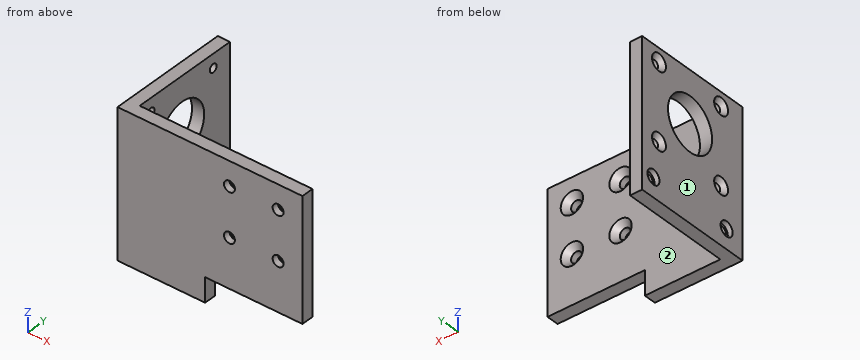
```python
from build123d import *

# Parameters (mm, degrees)
EXTRUDE_1_DEPTH             = 60
SKETCH_2_R                  = 11
CUT_EXTRUDE_1_DEPTH         = 60
CSK_1_D                     = 3.4
CSK_1_DEPTH                 = 5
CSK_1_CSINK_D               = 6.94
CSK_1_CSINK_ANGLE           = 90
SKETCH_5_W                  = 64
SKETCH_5_H                  = 10
CUT_EXTRUDE_2_DEPTH         = 127.885775404
SKETCH_6_R                  = 2
CUT_EXTRUDE_3_DEPTH         = 10
SKETCH_7_R                  = 3
CUT_EXTRUDE_4_DEPTH         = 2
SKETCH_8_W                  = 24
SKETCH_8_H                  = 50
CUT_EXTRUDE_5_DEPTH         = 127.885775404
HOLE_WIZARD_M41_D           = 4.5
HOLE_WIZARD_M41_CSINK_D     = 9.18
HOLE_WIZARD_M41_CSINK_ANGLE = 90


with BuildPart() as part:
    # Эскиз1 → Бобышка-Вытянуть1 (new body)
    with BuildSketch(Plane.XY):
        Polygon((0, 0), (0, 50), (5, 50), (5, 5), (95, 5), (95, 50), (100, 50), (100, 0), align=None)
    extrude(amount=EXTRUDE_1_DEPTH)

    # Эскиз2 → Вырез-Вытянуть1 (cut)
    with BuildSketch(Plane.ZY):
        with Locations((38.85, 26.15)):
            Circle(SKETCH_2_R)
    extrude(amount=-CUT_EXTRUDE_1_DEPTH, mode=Mode.SUBTRACT)

    # CSK размера винта с полупотайной головкой и крестообразным шлицем1
    with Locations(Plane.ZY):
        with Locations((54.35, 10.65), (54.35, 41.65), (23.35, 41.65), (23.35, 10.65)):
            CounterSinkHole(CSK_1_D / 2, CSK_1_CSINK_D / 2, depth=CSK_1_DEPTH, counter_sink_angle=CSK_1_CSINK_ANGLE)

    # Эскиз5 → Вырез-Вытянуть2 (cut, through all)
    with BuildSketch(Plane.XZ):
        with Locations((68, 5)):
            Rectangle(SKETCH_5_W, SKETCH_5_H)
    extrude(amount=-CUT_EXTRUDE_2_DEPTH, mode=Mode.SUBTRACT)

    # Эскиз6 → Вырез-Вытянуть3 (cut)
    with BuildSketch(Plane.ZY):
        with Locations((8, 44.4)):
            Circle(SKETCH_6_R)
        with Locations((8, 7.9)):
            Circle(SKETCH_6_R)
    extrude(amount=-CUT_EXTRUDE_3_DEPTH, mode=Mode.SUBTRACT)

    # Эскиз7 → Вырез-Вытянуть4 (cut)
    with BuildSketch(Plane.ZY):
        with Locations((8, 44.4)):
            Circle(SKETCH_7_R)
        with Locations((8, 7.9)):
            Circle(SKETCH_7_R)
    extrude(amount=-CUT_EXTRUDE_4_DEPTH, mode=Mode.SUBTRACT)

    # Эскиз8 → Вырез-Вытянуть5 (cut, through all)
    with BuildSketch(Plane.XZ):
        with Locations((88, 35)):
            Rectangle(SKETCH_8_W, SKETCH_8_H)
    extrude(amount=-CUT_EXTRUDE_5_DEPTH, mode=Mode.SUBTRACT)

    # Зенковка для винта с потайной головкой и внутренним шестигранником M41 (through all)
    with Locations(Plane(origin=(0, 5, 0), x_dir=(-1, 0, 0), z_dir=(0, 1, 0))):
        with Locations((-46, 30), (-66, 30), (-46, 50), (-66, 50)):
            CounterSinkHole(HOLE_WIZARD_M41_D / 2, HOLE_WIZARD_M41_CSINK_D / 2, counter_sink_angle=HOLE_WIZARD_M41_CSINK_ANGLE)


solid = part.part
```
Design review of the part built by this model. Coordinates are the model's own, in mm. Face numbers are marked on the shaded views. A direction names the side the tool comes from. Give positions to 0.01 mm unless a question says otherwise; leave off trailing zeros. Order: outer loops, then holes, each group sorted by start corner. A loop starts at its lowest first (then second) coordinate and runs counter-clockwise, first axis right, second up. Notation, with made-up numbers: (-23, 59) - (0, 59) arc R21 ccw to (0, 83) - close; hole circle Ø4 at (28.25, -24.75). An arc over 180 degrees is marked (long way). Use a Markdown table: item, result. Add a question column.
(1) Add section A-A on x = 66. Give the boundary of the cut face in (y, z).
(2) Add section C-C on z = 42. Give the boundary of the cut face in (x, y).
(3) Machinability: for the marked faces 1 and 2, which of the approach directions +Z, -Z, +X, -X, +Y, -Y give a long, thin tool a straight path to every point of the face, cutting with its end or side? Answer none if there is none.
(4) Wall thickness on probe 1 along Y at (x, z) = (1.2, 8); probe 2 along X at (y, z) = (2, 50); probe 3 along Y at (x, z) = (4.2, 8): over which ranges is each line inside the solid? List them lowest first. Write a range as [from, to].
(5) Add section B-B on z = 8. Give the boundary of the cut face in (x, y).
(6) Clearance check with flat-ended pins moving along their axes: P1, Ø17.5, axis at y = 26.15, z = 38.85, coming from the -X side; P2, Ø5, axis at y = 44.4, z = 8, coming from the +X side; P3, Ø4, axis at x = 24, z = 49.5, coming from the +Y side; P4, Ø3, axis at x = 65, z = 49.5, coming from the +Y side. State where each tip first meets the part, or that it passes through.
(7) Add section D-D on z = 17. Give the boundary of the cut face in (x, y).
Report:
| question | item | result |
|---|---|---|
| 1 | outline | (0, 10) - (5, 10) - (5, 25.41) - (2.66, 27.75) - (0, 27.75) - close; (0, 32.25) - (2.66, 32.25) - (5, 34.59) - (5, 45.41) - (2.66, 47.75) - (0, 47.75) - close; (0, 52.25) - (2.66, 52.25) - (5, 54.59) - (5, 60) - (0, 60) - close |
| 2 | outline | (0, 0) - (76, 0) - (76, 5) - (5, 5) - (5, 15.61) - (0, 15.61) - close; (0, 36.69) - (5, 36.69) - (5, 50) - (0, 50) - close |
| 3 | face 1 | +Z, -Z, -X, +Y, -Y |
| 3 | face 2 | +Z, -Z, +X, +Y |
| 4 | probe 1 | y = [0, 4.9], [10.9, 41.4], [47.4, 50] |
| 4 | probe 2 | x = [0, 43.75], [48.25, 63.75], [68.25, 76] |
| 4 | probe 3 | y = [0, 5.9], [9.9, 42.4], [46.4, 50] |
| 5 | outline | (0, 0) - (36, 0) - (36, 5) - (5, 5) - (5, 5.9) - (2, 5.9) - (2, 4.9) - (0, 4.9) - close; (0, 10.9) - (2, 10.9) - (2, 9.9) - (5, 9.9) - (5, 42.4) - (2, 42.4) - (2, 41.4) - (0, 41.4) - close; (0, 47.4) - (2, 47.4) - (2, 46.4) - (5, 46.4) - (5, 50) - (0, 50) - close |
| 6 | P1 | passes through |
| 6 | P2 | stops at x = 5 |
| 6 | P3 | stops at y = 5 |
| 6 | P4 | stops at y = 3.03 |
| 7 | outline | (0, 0) - (76, 0) - (76, 5) - (5, 5) - (5, 50) - (0, 50) - close |
